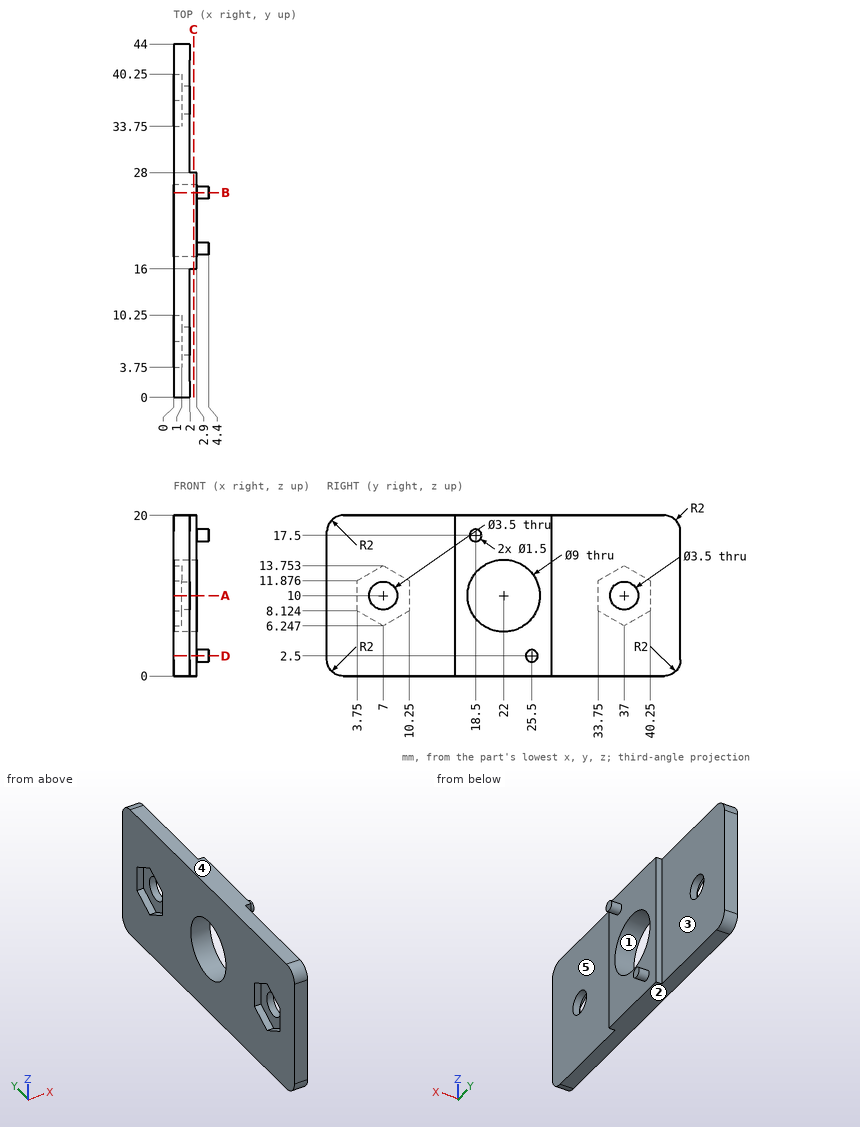
Design review of the part shown in the three views and the two pictorial views. Dimensions are in mm from the part's minimum x, y and z. A direction names the side the tool comes from. Give positions to 0.01 mm unless a question says otherwise; leave off trailing zeros. Order: outer loops, then holes, each group sorted by start corner. A loop starts at its lowest first (then second) coordinate and runs counter-clockwise, first axis right, second up. Notation, with made-up numbers: M -2,-38.5 L 52,-38.5 A14 ccw 52,-33.5 Z; hole C -12,39.25 d8. An arc over 180 degrees is marked long. Answer in a Markdown table with one row per item. Add a question column.
(1) Consider section D-D on z = 2.5. State the section outline as (x, y) points, and give its area (3 significant figures).
(2) Mouldability with a two-part tool opening along Y and no side actions: class the marked faces 1 and 2 as +Y half, -Y half, draft (parallel to the pull), parting line (faces both ways), or undercut.
(3) For pin 1 (12 mm diameter, centred on y = 34.5, z = 9.5, fed in from +X); pin 2 (3 mm diameter, centred on y = 7, z = 10.5, fed in from -X); pin 3 (2 mm diameter, centred on x = 3.5, z = 16.5, fed in from -Y); pin 4 (3 mm diameter, centred on y = 7, z = 10, fed in from +X), all flat-tipped, find the tip position at first contact; note any pin that passes through.
(4) Consider section A-A on z = 10. State the section outline as (x, y) points.
(5) Wall thickness on probe 1 along Y at (x, z) = (1.5, 10); probe 2 along Y at (x, z) = (2.8, 8.5); probe 3 along Y at (x, z) = (2.15, 10): over which ranges is each line inside the solid? List them lowest first. Write a range as [from, to].
(6) Consider section B-B on y = 25.5. State the section outline as (x, z) points.
(7) For the marked faces 3, 4 and 5, list the 3-axis set-ups (+Z, -Z, +X, -X, +Y, -Y) from which the entire face can be reached by the end or side of a thin tool; tool diameter is ignored.
(8) Consider section C-C on x = 2.5. State the section outline as (y, z) points, and give its area (3 significant figures).
Evaluation:
| question | item | result |
|---|---|---|
| 1 | outline | M 0,0 L 2,0 L 2,16 L 2.9,16 L 2.9,24.75 L 4.4,24.75 L 4.4,26.25 L 2.9,26.25 L 2.9,28 L 2,28 L 2,44 L 0,44 Z |
| 1 | area | 101 mm^2 |
| 2 | face 1 | undercut |
| 2 | face 2 | draft |
| 3 | pin 1 | stops at x = 2 |
| 3 | pin 2 | stops at x = 1 |
| 3 | pin 3 | stops at y = 16 |
| 3 | pin 4 | passes through |
| 4 | outline | M 0,0 L 2,0 L 2,5.25 L 1,5.25 L 1,3.75 L 0,3.75 Z; M 0,10.25 L 1,10.25 L 1,8.75 L 2,8.75 L 2,16 L 2.9,16 L 2.9,17.5 L 0,17.5 Z; M 0,26.5 L 2.9,26.5 L 2.9,28 L 2,28 L 2,35.25 L 1,35.25 L 1,33.75 L 0,33.75 Z; M 0,40.25 L 1,40.25 L 1,38.75 L 2,38.75 L 2,44 L 0,44 Z |
| 5 | probe 1 | y = [0, 5.25], [8.75, 17.5], [26.5, 35.25], [38.75, 44] |
| 5 | probe 2 | y = [16, 17.76], [26.24, 28] |
| 5 | probe 3 | y = [16, 17.5], [26.5, 28] |
| 6 | outline | M 0,0 L 2.9,0 L 2.9,1.75 L 4.4,1.75 L 4.4,3.25 L 2.9,3.25 L 2.9,7.17 L 0,7.17 Z; M 0,12.83 L 2.9,12.83 L 2.9,20 L 0,20 Z |
| 7 | face 3 | +Z, -Z, +X, +Y |
| 7 | face 4 | +Z, +X, -X, +Y, -Y |
| 7 | face 5 | +Z, -Z, +X, -Y |
| 8 | outline | M 16,0 L 28,0 L 28,20 L 16,20 Z; hole C 22,10 d9 |
| 8 | area | 176 mm^2 |
